```python
from build123d import *

# Parameters (mm, degrees)
BOSS_EXTRUDE1_DEPTH                               = 50.8
FILLET1_R                                         = 1.5875
SKETCH3_W                                         = 50.927
SKETCH3_H                                         = 3.175
BOSS_EXTRUDE2_DEPTH                               = 27.94
SKETCH4_W                                         = 44.577
SKETCH4_H                                         = 21.59
CUT_EXTRUDE1_DEPTH                                = 3.175
FILLET2_R                                         = 6.35
SKETCH6_W                                         = 1.016
SKETCH6_H                                         = 10.0076
BOSS_EXTRUDE3_DEPTH                               = 3.175
CSK_FOR_2_FLAT_HEAD_MACHINE_SCREW_100_D           = 2.7051
CSK_FOR_2_FLAT_HEAD_MACHINE_SCREW_100_CSINK_D     = 4.3688
CSK_FOR_2_FLAT_HEAD_MACHINE_SCREW_100_CSINK_ANGLE = 100


with BuildPart() as part:
    # Sketch1 → Boss-Extrude1 (new body)
    with BuildSketch(Plane.XY):
        Polygon((143.005117829, 31.115), (-32.877459737, -3.175), (248.569196095, -3.175), (195.170369003, 31.115), align=None)
        with BuildLine():
            Line((16.438729869, 0), (232.338729869, 0))
            ThreePointArc((232.338729869, 0), (233.862005994, 1.140525622), (233.196513049, 2.923300983))
            Line((233.196513049, 2.923300983), (194.238729869, 27.94))
            Line((194.238729869, 27.94), (143.311729869, 27.94))
            Line((143.311729869, 27.94), (16.134950843, 3.14566384))
            ThreePointArc((16.134950843, 3.14566384), (14.858580928, 1.434903877), (16.438729869, 0))
        make_face(mode=Mode.SUBTRACT)
    extrude(amount=BOSS_EXTRUDE1_DEPTH)

    # Fillet1
    fillet1_edges = [part.edges().sort_by_distance(p)[0] for p in [
        (195.170369003, 31.115, 25.4),
        (248.569196095, -3.175, 25.4),
        (-32.877459737, -3.175, 25.4),
        (143.005117829, 31.115, 25.4),
    ]]
    fillet(fillet1_edges, radius=FILLET1_R)

    # Sketch3 → Boss-Extrude2 (add)
    with BuildSketch(Plane.XZ.offset(-27.94)):
        with Locations((168.775229869, 25.4)):
            Rectangle(SKETCH3_W, SKETCH3_H)
    extrude(amount=BOSS_EXTRUDE2_DEPTH)

    # Sketch4 → Cut-Extrude1 (cut)
    with BuildSketch(Plane(origin=(0, 0, 23.8125), x_dir=(-1, 0, 0), z_dir=(0, 0, -1))):
        with Locations((-168.775229869, 13.97)):
            Rectangle(SKETCH4_W, SKETCH4_H)
    extrude(amount=-CUT_EXTRUDE1_DEPTH, mode=Mode.SUBTRACT)

    # Fillet2
    fillet2_edges = [part.edges().sort_by_distance(p)[0] for p in [
        (191.063729869, 24.765, 25.4),
        (146.486729869, 24.765, 25.4),
        (146.486729869, 3.175, 25.4),
        (191.063729869, 3.175, 25.4),
    ]]
    fillet(fillet2_edges, radius=FILLET2_R)

    # Sketch6 → Boss-Extrude3 (add)
    with BuildSketch(Plane.XY.offset(26.9875)):
        Polygon((143.311729869, 0), (140.136729869, 0), (140.136729869, 27.321003215), (143.311729869, 27.94), align=None)
        with Locations((141.724229869, 13.97)):
            Rectangle(SKETCH6_W, SKETCH6_H, mode=Mode.SUBTRACT)
    extrude(amount=-BOSS_EXTRUDE3_DEPTH)

    # CSK for #2 Flat Head Machine Screw (100)1 (through all)
    with Locations(Plane(origin=(0, 31.115, 0), x_dir=(1, 0, 0), z_dir=(0, 1, 0))):
        with Locations((155.858423849, -12.7), (182.004549436, -12.7), (182.004549436, -38.1), (155.858423849, -38.1)):
            CounterSinkHole(CSK_FOR_2_FLAT_HEAD_MACHINE_SCREW_100_D / 2, CSK_FOR_2_FLAT_HEAD_MACHINE_SCREW_100_CSINK_D / 2, counter_sink_angle=CSK_FOR_2_FLAT_HEAD_MACHINE_SCREW_100_CSINK_ANGLE)


solid = part.part
```
Model file for the job. Use its own axes, mm. A direction names the side the tool comes from. Coordinates: 2 decimals unless noted, no trailing zeros. Order: outer loops, then holes, each group sorted by start corner. A loop starts at its lowest first (then second) coordinate and runs counter-clockwise, first axis right, second up. Notation, with made-up numbers: (-8.75, 51) -> (13.25, 51) arc R19 ccw to (13.25, 84) -> close; hole circle Ø2 at (54, 75). An arc over 180 degrees is marked (long way). Return JSON: item names as keys, results as strings.
Item 1: Slice it at B-B (x = 171). Write the cut outline in (y, z) (1 decimal), then the cut area to 3 significant figures.
Model answer:
{"outline": "(-3.2, 0) -> (0, 0) -> (0, 23.8) -> (3.2, 23.8) -> (3.2, 27) -> (0, 27) -> (0, 50.8) -> (-3.2, 50.8) -> close; (24.8, 23.8) -> (27.9, 23.8) -> (27.9, 0) -> (31.1, 0) -> (31.1, 50.8) -> (27.9, 50.8) -> (27.9, 27) -> (24.8, 27) -> close", "area": "343 mm²"}
Item 2: Pin check, flat tips, straight feed: P1, Ø4, axis at y = 1, z = 36, coming from the +X side; P2, Ø1, axis at x = 141.5, y = 2, coming from the -Z side; P3, Ø8.5, axis at x = 169, y = 19.5, coming from the -Z side; P4, Ø1.6, axis at y = 11.5, z = 25, coming from the +X side. Stop position of each tip, or through.
Model answer:
{"P1": "stops at x = 244.63", "P2": "stops at z = 23.81", "P3": "passes through", "P4": "stops at x = 226.96"}
Item 3: 3-axis set-ups, long thin cutter, end or side, ignore diameter. For faces 1 (the face through (168, 2, 26.988)), 2 (the face through (169, 27.94, 12)), 3 (the face through (148.3, 5.08, 25.42)): which of +Z, -Z, +X, -X, +Y, -Y reach the whole face in a straight line?
Model answer:
{"face 1": "+Z", "face 2": "-Z", "face 3": "+Z, -Z"}
Item 4: Slice it at C-C (y = 13.5). Write the cut outline in (x, z).
Model answer:
{"outline": "(52.65, 0) -> (69.25, 0) -> (69.25, 50.8) -> (52.65, 50.8) -> close; (140.14, 23.81) -> (141.22, 23.81) -> (141.22, 26.99) -> (140.14, 26.99) -> close; (142.23, 23.81) -> (146.49, 23.81) -> (146.49, 26.99) -> (142.23, 26.99) -> close; (191.06, 23.81) -> (194.24, 23.81) -> (194.24, 26.99) -> (191.06, 26.99) -> close; (216.73, 0) -> (222.6, 0) -> (222.6, 50.8) -> (216.73, 50.8) -> close"}
Item 5: Wall check: line 1 along X through (y, z) = (-2.4, 38.1); line 2 along Y through (x, z) = (122, 44) (3 decimals); line 3 along X through (y, z) = (-1, 38). Give the ranges that are in metal, low to high. Write a range as from..to.
Model answer:
{"line 1": "x = -17.8..154.51, 157.21..180.65, 183.36..244.52", "line 2": "y = -3.175..0, 23.785..27.02", "line 3": "x = -17.91..154.51, 157.21..180.66, 183.35..244.63"}
Item 6: Slice it at D-D (x = 228.5). Write the cut outline in (y, z) (3 decimals).
Model answer:
{"outline": "(-3.175, 0) -> (0, 0) -> (0, 50.8) -> (-3.175, 50.8) -> close; (5.939, 0) -> (9.712, 0) -> (9.712, 50.8) -> (5.939, 50.8) -> close"}
